Work out the finished part from the listing and answer in its coordinate system (mm). A direction names the side the tool comes from. Give positions to 0.01 mm unless a question says otherwise; leave off trailing zeros. Loops run counter-clockwise (first coordinate to the right, second up) from the corner with the lowest first, then second, coordinate; pieces in that order, holes last. Notation, with made-up numbers: (43.5, 68.5) - (99.5, 68.5) arc R11 ccw to (99.5, 73.5) - close; hole circle Ø7 at (-34, 12.5). An arc over 180 degrees is marked (long way). Use CSV: the item, a comma, the result in double quotes.
from build123d import *

# Parameters (mm, degrees)
SKETCH1_R           = 17.5
SKETCH1_R_2         = 12
BOSS_EXTRUDE1_DEPTH = 21
SKETCH1_3_R         = 12
SKETCH1_3_R_2       = 7.5
BOSS_EXTRUDE2_DEPTH = 13
BOSS_EXTRUDE3_DEPTH = 9
BOSS_EXTRUDE4_DEPTH = 2.5


with BuildPart() as part:
    # Sketch1 → Boss-Extrude1 (new, symmetric)
    with BuildSketch(Plane(origin=(0, 0, 0), x_dir=(0, 1, 0), z_dir=(0, 0, 1))):
        with Locations(Location((0, 0, 0), (0, 0, 90))):
            Circle(SKETCH1_R)
        with Locations(Location((0, 0, 0), (0, 0, 90))):
            Circle(SKETCH1_R_2, mode=Mode.SUBTRACT)
    extrude(amount=BOSS_EXTRUDE1_DEPTH, both=True)



with BuildPart() as body_2:
    # Sketch1_3 → Boss-Extrude2 (new, symmetric)
    with BuildSketch(Plane(origin=(0, 0, 0), x_dir=(0, 1, 0), z_dir=(0, 0, 1))):
        with Locations(Location((178, 0, 0), (0, 0, 90))):
            Circle(SKETCH1_3_R)
        with Locations(Location((178, 0, 0), (0, 0, 90))):
            Circle(SKETCH1_3_R_2, mode=Mode.SUBTRACT)
    extrude(amount=BOSS_EXTRUDE2_DEPTH, both=True)


with BuildPart() as part_1:
    add(part.part)

    add(body_2.part)  # Boss-Extrude3 merges body 2
    # Sketch1_4 → Boss-Extrude3 (add, symmetric)
    with BuildSketch(Plane(origin=(0, 0, 0), x_dir=(0, 1, 0), z_dir=(0, 0, 1))):
        with BuildLine():
            Line((163.61250543, 9), (25.164459064, 9))
            ThreePointArc((25.164459064, 9), (17.484097627, 10.26210106), (10.611518883, 13.915662651))
            ThreePointArc((10.611518883, 13.915662651), (15.683615343, 7.76364668), (17.5, 0))
            ThreePointArc((17.5, 0), (15.683615343, -7.76364668), (10.611518883, -13.915662651))
            ThreePointArc((10.611518883, -13.915662651), (17.484097627, -10.26210106), (25.164459064, -9))
            Line((25.164459064, -9), (163.61250543, -9))
            ThreePointArc((163.61250543, -9), (168.511484916, -9.505319751), (173.204168477, -11))
            ThreePointArc((173.204168477, -11), (166, 0), (173.204168477, 11))
            ThreePointArc((173.204168477, 11), (168.511484916, 9.505319751), (163.61250543, 9))
        make_face()
        with BuildLine():
            ThreePointArc((24, -5), (19, 0), (24, 5))
            Line((24, 5), (154, 5))
            ThreePointArc((154, 5), (159, 0), (154, -5))
            Line((154, -5), (24, -5))
        make_face(mode=Mode.SUBTRACT)
    extrude(amount=BOSS_EXTRUDE3_DEPTH, both=True)

    # Sketch1_5 → Boss-Extrude4 (add, symmetric)
    with BuildSketch(Plane(origin=(0, 0, 0), x_dir=(0, 1, 0), z_dir=(0, 0, 1))):
        with BuildLine():
            Line((24, -5), (154, -5))
            ThreePointArc((154, -5), (159, 0), (154, 5))
            Line((154, 5), (24, 5))
            ThreePointArc((24, 5), (19, 0), (24, -5))
        make_face()
    extrude(amount=BOSS_EXTRUDE4_DEPTH, both=True)


solid = part_1.part
Item 1: A cutting plane is placed at B-B on x = 0. Determine the outline of the cut face in (y, z).
Determined:
outline,"(-17.5, -21) - (-12, -21) - (-12, 21) - (-17.5, 21) - close; (12, -21) - (17.5, -21) - (17.5, -9) - (19, -9) - (19, -2.5) - (159, -2.5) - (159, -9) - (166, -9) - (166, -13) - (170.5, -13) - (170.5, 13) - (166, 13) - (166, 9) - (159, 9) - (159, 2.5) - (19, 2.5) - (19, 9) - (17.5, 9) - (17.5, 21) - (12, 21) - close; (185.5, -13) - (190, -13) - (190, 13) - (185.5, 13) - close"
Item 2: For faces 4 (the cylindrical face through (-10.227, 17.588, 0.126)), 5 (the cylindrical face through (0, 159, -6)), 6 (the flat face through (6, 183, 13)), 7 (the flat face through (6, 183, -13)), determine the directions among +Z, -Z, +X, -X, +Y, -Y from which every point of the face is accessible in a straight line to the end or side of a thin tool.
Determined:
face 4,"+Z, -Z, -X"
face 5,"-Z"
face 6,"+Z, +X, -X, +Y"
face 7,"-Z, +X, -X, +Y"
Item 3: A cutting plane is placed at A-A on y = 0. Determine the outline of the cut face in (x, z).
Determined:
outline,"(-17.5, -21) - (-12, -21) - (-12, 21) - (-17.5, 21) - close; (12, -21) - (17.5, -21) - (17.5, 21) - (12, 21) - close"
Item 4: The mould has two halves that part along Y. Classify faces 1 (the cylindrical face through (-9.52, 168.58, 0.13)), 2 (the flat face through (12, 4, -21)), 3 (the cylindrical face through (2.601, 189.715, 0.182)): pulls with the +Y half, pulls with the -Y half, needs draft (parallel to the pull), parting line crosses it, or undercut.
Determined:
face 1,"undercut"
face 2,"needs draft"
face 3,"undercut"
Item 5: Find the intervals of material crossed by line 1 (Y direction, x = 0, z = 0); line 2 (Y direction, x = 0, z = 4.5); line 3 (Y direction, x = 0, z = 12), in increasing order.
Determined:
line 1,"y = -17.5 to -12, 12 to 170.5, 185.5 to 190"
line 2,"y = -17.5 to -12, 12 to 19, 159 to 170.5, 185.5 to 190"
line 3,"y = -17.5 to -12, 12 to 17.5, 166 to 170.5, 185.5 to 190"
Item 6: A cutting plane is placed at C-C on z = 0.5. Determine the outline of the cut face in (x, y), and give its area (3 significant figures).
Determined:
outline,"(-13.92, 10.61) arc R17.5 ccw (long way) to (13.92, 10.61) arc R24 cw to (9, 25.16) - (9, 163.61) arc R24 cw to (11, 173.2) arc R12 ccw (long way) to (-11, 173.2) arc R24 cw to (-9, 163.61) - (-9, 25.16) arc R24 cw to start; hole circle Ø24 at (0, 0); hole circle Ø15 at (0, 178)"
area,"3,520 mm²"
Item 7: Given P1, Ø12, axis at x = 0, y = 173, coming from the -Z side; P2, Ø5.5, axis at y = 79.5, z = 1.5, coming from the +X side; P3, Ø1, axis at x = 13, z = -13, coming from the +Y side, each flat-ended and moving along its own axis, determine where each tip first touches the part or whether it passes through.
Determined:
P1,"stops at z = -13"
P2,"stops at x = 9"
P3,"stops at y = 12.25"
Item 8: A cutting plane is placed at D-D on y = 74. Determine the outline of the cut face in (x, z).
Determined:
outline,"(-9, -9) - (-5, -9) - (-5, -2.5) - (5, -2.5) - (5, -9) - (9, -9) - (9, 9) - (5, 9) - (5, 2.5) - (-5, 2.5) - (-5, 9) - (-9, 9) - close"
